The listing builds one solid part. Answer for the finished solid, in the listing's coordinates (mm). Round coordinates to 2 decimals unless told otherwise and drop trailing zeros. Loops run counter-clockwise (first coordinate to the right, second up) from the corner with the lowest first, then second, coordinate; pieces in that order, holes last. Notation, with made-up numbers: (-15, -39) -> (12, -39) arc R15 cw to (12, -16) -> close; hole circle Ø6 at (82, 52.5). An arc over 180 degrees is marked (long way). Use a Markdown table: item, result. Add a question column.
Q1. Given pin 1 Ø1.9 at (x, z) = (-20, 65) entering from +Y; pin 2 Ø5 at (x, z) = (-40, -40) entering from -Y, each flat-ended and moving along its own axis, determine where each tip first touches the part or whether it passes through.
Q2. Consider line 1 (X direction, y = 1.9, z = -40); line 2 (X direction, y = 1.25, z = 103.95); line 3 (X direction, y = 1.55, z = 78.95). Determine where each line is inside the solid, lowest interval first.
Q3. Section A-A on y = 1.9 is taken. Give the number of separate pieces and of enclosed holes in the cut face, then the cut area to 3 significant figures.
Q4. Section B-B on x = -11.5 is taken. Give the vertices of the cut face in (y, z), then the cut area to 3 significant figures.
from build123d import *

# Parameters (mm, degrees)
SKETCH_1_W          = 105
SKETCH_1_H          = 271
EXTRUDE_1_DEPTH     = 2.5
SKETCH_2_R          = 1.6
CUT_EXTRUDE_1_DEPTH = 10
CHAMFER_4_SIZE      = 1.4
CHAMFER_5_SIZE      = 1
CUT_EXTRUDE_2_DEPTH = 10
SKETCH_6_R          = 1.6
CUT_EXTRUDE_3_DEPTH = 10
SKETCH_7_R          = 1.6
CUT_EXTRUDE_4_DEPTH = 10
SKETCH_8_R          = 1.6
CUT_EXTRUDE_5_DEPTH = 10
SKETCH_9_R          = 2
CUT_EXTRUDE_6_DEPTH = 10
CHAMFER_3_SIZE      = 1.2


with BuildPart() as part:
    # 草图1 → 凸台-拉伸1 (new body)
    with BuildSketch(Plane(origin=(0, 0, 0), x_dir=(1, 0, 0), z_dir=(0, 1, 0))):
        Rectangle(SKETCH_1_W, SKETCH_1_H)
    extrude(amount=EXTRUDE_1_DEPTH)

    # 草图2 → 切除-拉伸1 (cut)
    with BuildSketch(Plane(origin=(0, 2.5, 0), x_dir=(1, 0, 0), z_dir=(0, 1, 0))):
        with Locations((35, -3.95)):
            Circle(SKETCH_2_R)
        with Locations((13.000000181, -3.95)):
            Circle(SKETCH_2_R)
        with Locations((35, -78.95)):
            Circle(SKETCH_2_R)
        with Locations((13.000000181, -78.95)):
            Circle(SKETCH_2_R)
        with Locations((20, -35)):
            Circle(SKETCH_2_R)
        with Locations((-20, -35)):
            Circle(SKETCH_2_R)
        with Locations((20, -65)):
            Circle(SKETCH_2_R)
        with Locations((-20, -65)):
            Circle(SKETCH_2_R)
        with Locations((-20, 35)):
            Circle(SKETCH_2_R)
        with Locations((20, 35)):
            Circle(SKETCH_2_R)
        with Locations((-20, 65)):
            Circle(SKETCH_2_R)
        with Locations((20, 65)):
            Circle(SKETCH_2_R)
    extrude(amount=-CUT_EXTRUDE_1_DEPTH, mode=Mode.SUBTRACT)

    # 倒角4
    chamfer_4_edges = [part.edges().sort_by_distance(p)[0] for p in [
        (-21.6, 2.5, 35),
        (18.4, 2.5, 65),
        (-21.6, 2.5, 65),
        (-21.6, 2.5, -35),
        (18.4, 2.5, 35),
        (18.4, 2.5, -65),
        (-21.6, 2.5, -65),
        (18.4, 2.5, -35),
    ]]
    chamfer(chamfer_4_edges, length=CHAMFER_4_SIZE)

    # 倒角5
    chamfer_5_edges = [part.edges().sort_by_distance(p)[0] for p in [
        (-52.5, 0, 0),
        (52.5, 0, 0),
    ]]
    chamfer(chamfer_5_edges, length=CHAMFER_5_SIZE)

    # 草图4 → 切除-拉伸2 (cut)
    with BuildSketch(Plane.XZ):
        Polygon((0, 100.95), (22.5, 100.95), (22.5, 135.5), (-22.5, 135.5), (-22.5, 100.95), align=None)
        Polygon((-22.5, -100.95), (0, -100.95), (22.5, -100.95), (22.5, -135.5), (-22.5, -135.5), align=None)
    extrude(amount=-CUT_EXTRUDE_2_DEPTH, mode=Mode.SUBTRACT)

    # 草图6 → 切除-拉伸3 (cut)
    with BuildSketch(Plane.XZ):
        with Locations((-40, 132.5)):
            Circle(SKETCH_6_R)
        with Locations((-30, 132.5)):
            Circle(SKETCH_6_R)
        with Locations((-30, 103.95)):
            Circle(SKETCH_6_R)
        with Locations((-40, 103.95)):
            Circle(SKETCH_6_R)
        with Locations((40, 103.95)):
            Circle(SKETCH_6_R)
        with Locations((30, 103.95)):
            Circle(SKETCH_6_R)
        with Locations((30, 132.5)):
            Circle(SKETCH_6_R)
        with Locations((40, 132.5)):
            Circle(SKETCH_6_R)
        with Locations((40, -132.5)):
            Circle(SKETCH_6_R)
        with Locations((30, -132.5)):
            Circle(SKETCH_6_R)
        with Locations((30, -103.95)):
            Circle(SKETCH_6_R)
        with Locations((40, -103.95)):
            Circle(SKETCH_6_R)
        with Locations((-40, -103.95)):
            Circle(SKETCH_6_R)
        with Locations((-30, -103.95)):
            Circle(SKETCH_6_R)
        with Locations((-30, -132.5)):
            Circle(SKETCH_6_R)
        with Locations((-40, -132.5)):
            Circle(SKETCH_6_R)
    extrude(amount=-CUT_EXTRUDE_3_DEPTH, mode=Mode.SUBTRACT)

    # 草图7 → 切除-拉伸4 (cut)
    with BuildSketch(Plane(origin=(0, 2.5, 0), x_dir=(1, 0, 0), z_dir=(0, 1, 0))):
        with Locations((-40, 60)):
            Circle(SKETCH_7_R)
        with Locations((-30, 60)):
            Circle(SKETCH_7_R)
        with Locations((30, 60)):
            Circle(SKETCH_7_R)
        with Locations((40, 60)):
            Circle(SKETCH_7_R)
        with Locations((-40, 40)):
            Circle(SKETCH_7_R)
        with Locations((-30, 40)):
            Circle(SKETCH_7_R)
        with Locations((30, 40)):
            Circle(SKETCH_7_R)
        with Locations((40, 40)):
            Circle(SKETCH_7_R)
    extrude(amount=-CUT_EXTRUDE_4_DEPTH, mode=Mode.SUBTRACT)

    # 草图8 → 切除-拉伸5 (cut)
    with BuildSketch(Plane.XZ):
        with Locations((-40, 84.45)):
            Circle(SKETCH_8_R)
        with Locations((-30, 84.45)):
            Circle(SKETCH_8_R)
        with Locations((-30, -13.05)):
            Circle(SKETCH_8_R)
        with Locations((-40, -13.05)):
            Circle(SKETCH_8_R)
    extrude(amount=-CUT_EXTRUDE_5_DEPTH, mode=Mode.SUBTRACT)

    # 草图9 → 切除-拉伸6 (cut)
    with BuildSketch(Plane.XZ):
        with Locations((20.5, 100.95)):
            Circle(SKETCH_9_R)
        with Locations((-20.5, 100.95)):
            Circle(SKETCH_9_R)
        with Locations((-20.5, -100.95)):
            Circle(SKETCH_9_R)
        with Locations((20.5, -100.95)):
            Circle(SKETCH_9_R)
    extrude(amount=-CUT_EXTRUDE_6_DEPTH, mode=Mode.SUBTRACT)

    # 倒角3
    chamfer_3_edges = [part.edges().sort_by_distance(p)[0] for p in [
        (28.4, 0, -40),
        (-31.6, 0, -60),
        (38.4, 0, -60),
        (-41.6, 0, -60),
        (-31.6, 0, -40),
        (38.4, 0, -40),
        (-41.6, 0, -40),
        (28.4, 0, -60),
        (-41.6, 0, -13.05),
        (-31.6, 0, -13.05),
        (-31.6, 0, 84.45),
        (-41.6, 0, 84.45),
        (11.400000181, 0, 3.95),
        (33.4, 0, 78.95),
        (11.400000181, 0, 78.95),
        (33.4, 0, 3.95),
    ]]
    chamfer(chamfer_3_edges, length=CHAMFER_3_SIZE)


solid = part.part
Checked values:
| question | item | result |
|---|---|---|
| 1 | pin 1 | passes through |
| 1 | pin 2 | stops at y = 0.3 |
| 2 | line 1 | x = -52.5 to -41.6, -38.4 to -31.6, -28.4 to 28.4, 31.6 to 38.4, 41.6 to 52.5 |
| 2 | line 2 | x = -52.5 to -41.6, -38.4 to -31.6, -28.4 to -22.5, 22.5 to 28.4, 31.6 to 38.4, 41.6 to 52.5 |
| 2 | line 3 | x = -52.5 to 11.4, 14.6 to 33.4, 36.6 to 52.5 |
| 3 | separate pieces | 1 |
| 3 | enclosed holes | 40 |
| 3 | area | 24,900 mm2 |
| 4 | outline | (0, -100.95) -> (2.5, -100.95) -> (2.5, 100.95) -> (0, 100.95) -> close |
| 4 | area | 505 mm2 |
